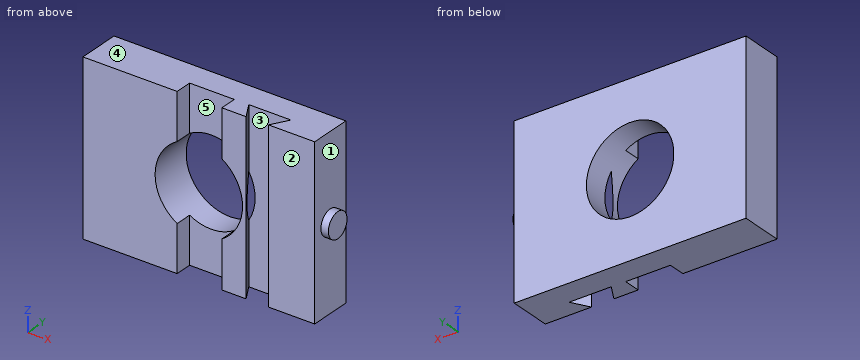
```python
from build123d import *

# Parameters (mm, degrees)
F0_W     = 69.9034725258
F0_H     = 50.9537383914
F0_R     = 13.1910844609
F1_DEPTH = 12.7
F3_DEPTH = 5.08
F5_DEPTH = 50.9547383914
F6_R     = 3.81
F7_DEPTH = 2.2606


with BuildPart() as f1:
    # F0 (on Front) → F1 (new body)
    with BuildSketch(Plane.XZ):
        with Locations((-0.2105524327, 0)):
            Rectangle(F0_W, F0_H)
        with Locations((-0.2105524327, 0)):
            Circle(F0_R, mode=Mode.SUBTRACT)
    extrude(amount=F1_DEPTH)

    # F2 (on face) → F3 (cut)
    with BuildSketch(Plane.XZ.offset(12.7)):
        with BuildLine():
            Line((6.7376832012, 25.4768691957), (-6.7376843654, 25.4768691957))
            Line((-6.7376843654, 25.4768691957), (-6.7376843654, 11.4630387764))
            ThreePointArc((-6.7376843654, 11.4630387764), (0.0343716306, 13.1888104641), (6.7376832012, 11.2127931771))
            Line((6.7376832012, 11.2127931771), (6.7376832012, 25.4768691957))
        make_face()
        with BuildLine():
            ThreePointArc((6.7376832012, -11.2127931771), (0.0343716306, -13.1888104641), (-6.7376843654, -11.4630387764))
            Line((-6.7376843654, -11.4630387764), (-6.7376843654, -25.4768691957))
            Line((-6.7376843654, -25.4768691957), (6.7376832012, -25.4768691957))
            Line((6.7376832012, -25.4768691957), (6.7376832012, -11.2127931771))
        make_face()
    extrude(amount=-F3_DEPTH, mode=Mode.SUBTRACT)

    # F4 (on face) → F5 (cut, through all)
    with BuildSketch(Plane(origin=(0, 0, -25.4768691957), x_dir=(1, 0, 0), z_dir=(0, 0, -1))):
        Polygon((20.8039732322, 12.7), (14.0363142386, 12.7), (11.0701437354, 7.5624419846), (23.7701437354, 7.5624419846), align=None)
    extrude(amount=-F5_DEPTH, mode=Mode.SUBTRACT)

    # F6 (on face) → F7 (join)
    with BuildSketch(Plane.YZ.offset(34.7411838302)):
        with Locations((-6.35, 0)):
            Circle(F6_R)
    extrude(amount=F7_DEPTH)


solid = f1.part
```
Source: CAD feature listing. Evaluate the final solid. Frame: model axes, mm. Face numbers are marked on the shaded views. A direction names the side the tool comes from. Give positions to 0.01 mm unless a question says otherwise; leave off trailing zeros. Order: outer loops, then holes, each group sorted by start corner. A loop starts at its lowest first (then second) coordinate and runs counter-clockwise, first axis right, second up.
(1) Contact query for flat-ended pins moving along their axis: P1, Ø4, axis at y = -2.5, z = -15, coming from the +X side; P2, Ø4, axis at x = -3.5, z = 21.5, coming from the -Y side. Output: stop coordinate, or through.
(2) Section query D-D (z = -18). Return the cut outline in (x, y), plus the area to 3 significant figures.
(3) Material intervals for line 1 along X through (y, z) = (-4, 0); line 2 along X through (y, z) = (-2.25, 0); line 3 along X through (y, z) = (-1.5, -19), sorted ascending.
(4) Section query A-A (y = -6.35). Return the cut outline in (x, z).
(5) Section query B-B (x = 4). Return the cut outline in (y, z), plus the area to 3 significant figures.
(6) Section query C-C (z = 0). Return the cut outline in (x, y).
(7) Pull-direction query (X, two-part tool) for the marked faces 1, 2 and 3; classes: +X half, -X half, draft (parallel to the pull), parting line (faces both ways), or undercut.
(8) Access query for the marked faces 4 and 5. Directions: +Z, -Z, +X, -X, +Y, -Y. A direction counts if a zero-diameter tool reaches every point of the face in a straight line with its end or side. Return the directions, or none.
Outcome:
1. P1: stops at x = 34.74
1. P2: stops at y = -7.62
2. outline: (-35.16, -12.7) - (-6.74, -12.7) - (-6.74, -7.62) - (6.74, -7.62) - (6.74, -12.7) - (14.04, -12.7) - (11.07, -7.56) - (23.77, -7.56) - (20.8, -12.7) - (34.74, -12.7) - (34.74, 0) - (-35.16, 0) - close
2. area: 769 mm2
3. line 1: x = -35.16 to -13.4, 12.98 to 37
3. line 2: x = -35.16 to -13.4, 12.98 to 34.74
3. line 3: x = -35.16 to 34.74
4. outline: (-35.16, -25.48) - (34.74, -25.48) - (34.74, -3.81) - (37, -3.81) - (37, 3.81) - (34.74, 3.81) - (34.74, 25.48) - (-35.16, 25.48) - close; hole circle Ø26.38 at (-0.21, 0)
5. outline: (-7.62, -25.48) - (0, -25.48) - (0, -12.5) - (-7.62, -12.5) - close; (-7.62, 12.5) - (0, 12.5) - (0, 25.48) - (-7.62, 25.48) - close
5. area: 198 mm2
6. outline: (-35.16, -12.7) - (-13.4, -12.7) - (-13.4, 0) - (-35.16, 0) - close; (12.98, -12.7) - (14.04, -12.7) - (12.98, -10.87) - close; (12.98, -7.56) - (23.77, -7.56) - (20.8, -12.7) - (34.74, -12.7) - (34.74, -10.16) - (37, -10.16) - (37, -2.54) - (34.74, -2.54) - (34.74, 0) - (12.98, 0) - close
7. face 1: +X half
7. face 2: draft
7. face 3: undercut
8. face 4: +Z, +X, -X, +Y, -Y
8. face 5: +Z, -Z, -Y
